```python
from build123d import *

# Parameters (mm, degrees)
F0_W     = 2000
F0_H     = 900
F1_DEPTH = 300
F2_R     = 50
F3_W     = 100
F3_H     = 100
F4_DEPTH = 300


with BuildPart() as f1:
    # F0 (on Top) → F1 (new body)
    with BuildSketch(Plane.XY):
        Rectangle(F0_W, F0_H)
    extrude(amount=F1_DEPTH)

    # F2
    f2_edges = [f1.edges().sort_by_distance(p)[0] for p in [
        (1000, 0, 300),
        (0, 450, 300),
        (-1000, 0, 300),
        (0, -450, 300),
        (-1000, -450, 150),
        (1000, -450, 150),
        (1000, 450, 150),
        (-1000, 450, 150),
    ]]
    fillet(f2_edges, radius=F2_R)

    # F3 (on face) → F4 (join)
    with BuildSketch(Plane(origin=(0, 0, 0), x_dir=(1, 0, 0), z_dir=(0, 0, -1))):
        with Locations((-850, 300)):
            Rectangle(F3_W, F3_H)
        with Locations((850, 300)):
            Rectangle(F3_W, F3_H)
        with Locations((-850, -300)):
            Rectangle(F3_W, F3_H)
        with Locations((850, -300)):
            Rectangle(F3_W, F3_H)
    extrude(amount=F4_DEPTH)


solid = f1.part
```
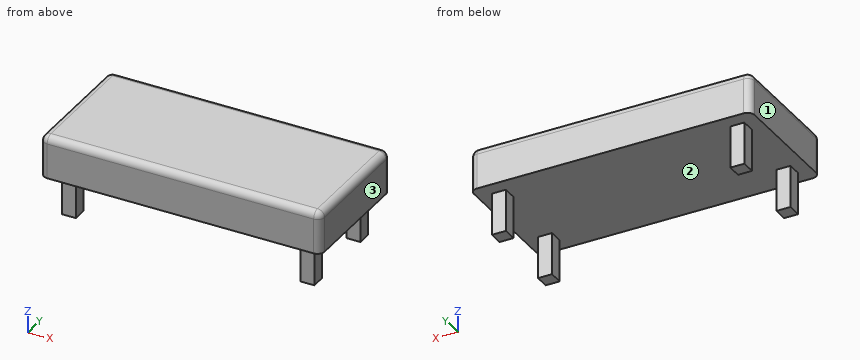
Geometry check sheet. Reference: the model listing, model coordinates, mm. Face numbers are marked on the shaded views. Coordinates: 2 decimals unless noted, no trailing zeros. Loops run counter-clockwise (first coordinate to the right, second up) from the corner with the lowest first, then second, coordinate; pieces in that order, holes last.
Item 1: Sectioned sample at C-C, the plane x = -857. Record the boundary of the cut face in (y, z).
Item 2: Sectioned sample at A-A, the plane y = 289. Record the boundary of the cut face in (x, z).
Item 3: Release check for a two-part mould opening along X. For the marked faces 1, 2 and 3 record: released by +X, released by -X, zero draft, split by the parting line, or undercut.
Item 4: Sectioned sample at B-B, the plane z = -92.5. Record the boundary of the cut face in (x, y).
Item 5: Thickness scan on line 1 (Z direction, x = -354.5, y = 128.5); line 2 (X direction, y = 115.5, z = 268); line 3 (Y direction, x = 759.5, z = 264). Record the ranges inside material, lowest first.
Item 6: Sectioned sample at D-D, the plane y = -380. Record the boundary of the cut face in (x, z), then the cut area to 3 significant figures.
Item 7: Go/stop test with a flat-tipped pin: pin 1 Ø6 at (x, y) = (412.5, 351) entering from -Z. Record where the tip stops, or that it passes through.
Check result:
1. outline: (-450, 0) - (-350, 0) - (-350, -300) - (-250, -300) - (-250, 0) - (250, 0) - (250, -300) - (350, -300) - (350, 0) - (450, 0) - (450, 250) arc R50 ccw to (400, 300) - (-400, 300) arc R50 ccw to (-450, 250) - close
2. outline: (-1000, 0) - (-900, 0) - (-900, -300) - (-800, -300) - (-800, 0) - (800, 0) - (800, -300) - (900, -300) - (900, 0) - (1000, 0) - (1000, 250) arc R50 ccw to (950, 300) - (-950, 300) arc R50 ccw to (-1000, 250) - close
3. face 1: released by -X
3. face 2: undercut
3. face 3: released by +X
4. outline: (-900, -350) - (-800, -350) - (-800, -250) - (-900, -250) - close; (-900, 250) - (-800, 250) - (-800, 350) - (-900, 350) - close; (800, -350) - (900, -350) - (900, -250) - (800, -250) - close; (800, 250) - (900, 250) - (900, 350) - (800, 350) - close
5. line 1: z = 0 to 300
5. line 2: x = -996.65 to 996.65
5. line 3: y = -448 to 448
6. outline: (-1000, 0) - (1000, 0) - (1000, 250) arc R50 ccw to (950, 300) - (-950, 300) arc R50 ccw to (-1000, 250) - close
6. area: 599,000 mm2
7. pin 1: stops at z = 0
